Build history of the part. All positions in model axes, mm. A direction names the side the tool comes from. Coordinates: 2 decimals unless noted, no trailing zeros. Order: outer loops, then holes, each group sorted by start corner. A loop starts at its lowest first (then second) coordinate and runs counter-clockwise, first axis right, second up. Notation, with made-up numbers: M 40,-33 L 65,-33 A18 ccw 65,-28 Z; hole C -38,-22.5 d11. An arc over 180 degrees is marked long. Write item = value, one per line. Start each with the question number.
Q1. Band-saw the part on C-C on y = 1.25. Write the cut outline in (x, z), plus the area to 3 significant figures.
Q2. Drill centre lines: probe 1 along Y at (x, z) = (-3, 21); probe 2 along Z at (x, y) = (-7, -0.5); probe 3 along X at (y, z) = (18.5, 4). Where is each one in solid material? Low to high.
Q3. Pull direction X, two halves, no side cores. Call faces 5 (the face through (6.73, 18.1, 27.31)), 6 (the face through (12.626, 11, -5)), 7 (the face through (3, -4.786, 8)), 8 (the face through (-7.574, 8, 8)): released by +X, released by -X, zero draft, split by the parting line, or undercut.
Q4. Band-saw the part on B-B on z = 23. Write the cut outline in (x, y).
Q5. 3-axis set-ups, long thin cutter, end or side, ignore diameter. For faces 1 (the face through (3, -6.786, -1)), 2 (the face through (9, 6.958, 22)), 3 (the face through (13.626, 8, 8)), 4 (the face through (-0.95, 18.09, 27.31)): which of +Z, -Z, +X, -X, +Y, -Y reach the whole face in a straight line?
Q6. Pin check, flat tips, straight feed: P1, Ø5.5, axis at y = 6.5, z = -4.5, coming from the +X side; P2, Ø5, axis at x = 8, z = 10.5, coming from the +Y side; P3, Ø2, axis at y = -2.5, z = 14, coming from the +X side; P4, Ø1.1, axis at y = 18.5, z = 22, coming from the -X side. Stop position of each tip, or through.
Q7. Band-saw the part on D-D on x = 5.25. Write the cut outline in (y, z).
Q8. Band-saw the part on A-A on x = -3. Write the cut outline in (y, z), plus the area to 3 significant figures.
Autodesk Inventor part; units mm, degrees
ref_plane "Płaszczyzna konstrukcyjna1" through (12.6265, -6.7865, 0) normal (1, 0, 0) x (0, 0, -1)
ref_plane "YZ Plane" through (0, 0, 0) normal (1, 0, 0) x (0, 1, 0)
ref_plane "XZ Plane" through (0, 0, 0) normal (0, 1, 0) x (-1, 0, 0)
sketch "Szkic1" plane through (0, 0, 0) normal (0, 0, 1) x (1, 0, 0)
  line L0 (-7.5735, 20.8135) -> (13.6265, 20.8135)
  line L1 (13.6265, 20.8135) -> (13.6265, -4.7865)
  line L2 (13.6265, -4.7865) -> (-7.5735, -4.7865)
  line L3 (-7.5735, -4.7865) -> (-7.5735, 20.8135)
  line L4 (-9.5735, 22.8135) -> (15.6265, 22.8135)
  line L5 (15.6265, 22.8135) -> (15.6265, -6.7865)
  line L6 (15.6265, -6.7865) -> (-9.5735, -6.7865)
  line L7 (-9.5735, -6.7865) -> (-9.5735, 22.8135)
  point P0 (0, 0)
  dimension "d0" = 21.2
  dimension "d1" = 25.6
  dimension "d2" = 2
extrude "Wyciągnięcie proste1" add sketch "Szkic1" along normal blind 16.3 contours L0 L1 L2 L3
extrude "Wyciągnięcie proste2" add sketch "Szkic1" against normal blind 2 contours L0 L1 L2 L3 | L4 L5 L6 L7
ref_plane "Płaszczyzna konstrukcyjna1" through (12.6265, -6.7865, 0) normal (1, 0, 0) x (0, 0, -1)
sketch "Szkic2" plane through (12.6265, -6.7865, 0) normal (1, 0, 0) x (0, 0, -1)
  line L0 (2, 0) -> (2, 29.6)
  line L1 (0, 0) -> (2, 0)
  line L2 (0, 29.6) -> (2, 29.6)
  line L3 (0, 27.6) -> (-16.3, 27.6)
  line L4 (0, 2) -> (-16.3, 2)
  arc A0 (9, 19.6) -> (2, 26.6) centre (-7.5761, 10.0239) ccw
  line L5 (9, 19.6) -> (2, 3)
  point P0 (0, 6.7865)
  dimension "d8" = 7
  dimension "d9" = 29.6
  dimension "d10" = 2
  dimension "d11" = 10
  dimension "d12" = 1
  dimension "d13" = 1
extrude "Wyciągnięcie proste3" add sketch "Szkic2" against normal blind 18.7
sketch "Szkic3" plane through (0, 0, 16.3) normal (0, 0, 1) x (1, 0, 0)
  line L0 (13.6265, 20.8135) -> (-7.5735, 20.8135)
  line L1 (-7.5735, 20.8135) -> (-7.5735, -4.7865)
  line L2 (-7.5735, -4.7865) -> (13.6265, -4.7865)
  line L3 (13.6265, -4.7865) -> (13.6265, 20.8135)
  line L4 (-5.9377, 18.5947) -> (0.0623, 18.5947)
  line L5 (0.0623, 18.5947) -> (0.0623, 17.5947)
  line L6 (0.0623, 17.5947) -> (-5.9377, 17.5947)
  line L7 (-5.9377, 17.5947) -> (-5.9377, 18.5947)
  line L8 (5.7192, 18.5947) -> (11.7192, 18.5947)
  line L9 (11.7192, 18.5947) -> (11.7192, 17.5947)
  line L10 (11.7192, 17.5947) -> (5.7192, 17.5947)
  line L11 (5.7192, 17.5947) -> (5.7192, 18.5947)
  line L12 (-5.9377, 7.9577) -> (0.0623, 7.9577)
  line L13 (0.0623, 7.9577) -> (0.0623, 6.9577)
  line L14 (0.0623, 6.9577) -> (-5.9377, 6.9577)
  line L15 (-5.9377, 6.9577) -> (-5.9377, 7.9577)
  line L16 (5.7192, 7.9577) -> (11.7192, 7.9577)
  line L17 (11.7192, 7.9577) -> (11.7192, 6.9577)
  line L18 (11.7192, 6.9577) -> (5.7192, 6.9577)
  line L19 (5.7192, 6.9577) -> (5.7192, 7.9577)
  point P0 (0, 0)
  dimension "d16" = 6
  dimension "d17" = 1
  dimension "d18" = 6
  dimension "d19" = 1
  dimension "d20" = 6
  dimension "d21" = 1
  dimension "d22" = 6
  dimension "d23" = 1
extrude "Wyciągnięcie proste4" add sketch "Szkic3" along normal blind 12 contours L4 L5 L6 L7 | L8 L9 L10 L11 | L12 L13 L14 L15 | L16 L17 L18 L19
chamfer "Faza1" distance 2 angle 45 8 edges at (0.0623, 18.0947, 28.3) (-5.9377, 18.0947, 28.3) (11.7192, 18.0947, 28.3) (5.7192, 18.0947, 28.3) (11.7192, 7.4577, 28.3) (5.7192, 7.4577, 28.3) (0.0623, 7.4577, 28.3) (-5.9377, 7.4577, 28.3)
sketch "Szkic4" plane through (12.6265, -3.7865, -2) normal (0, -0.3886, -0.9214) x (-1, 0, 0)
  line L0 (6.8473, 17.5297) -> (14.0234, 17.5297) construction
  line L1 (14.0234, 17.5297) -> (14.0234, 9.4771) construction
  line L2 (14.0234, 9.4771) -> (6.8473, 9.4771) construction
  line L3 (6.8473, 9.4771) -> (6.8473, 17.5297) construction
  line L4 (8.3846, 8.6266) -> (9.6316, 8.6266) construction
  line L5 (9.6316, 8.6266) -> (9.6316, 4.3438) construction
  line L6 (9.6316, 4.3438) -> (8.3846, 4.3438) construction
  line L7 (8.3846, 4.3438) -> (8.3846, 8.6266) construction
properties part number "COTS_GENERIC_AC_Power_Switch_10A"
Recorded:
q1.outline = M -9.57,-2 L -6.07,-2 L -6.07,-4.12 L 12.63,-4.12 L 12.63,-2 L 15.63,-2 L 15.63,0 L 13.63,0 L 13.63,16.3 L -7.57,16.3 L -7.57,0 L -9.57,0 Z
q1.area = 436 mm2
q2.probe_1 = 6.96 to 7.96, 17.59 to 18.59
q2.probe_2 = -2 to 16.3
q2.probe_3 = -7.57 to 13.63
q3.face_5 = undercut
q3.face_6 = released by +X
q3.face_7 = zero draft
q3.face_8 = released by -X
q4.outline = M -5.94,6.96 L 0.06,6.96 L 0.06,7.96 L -5.94,7.96 Z; M -5.94,17.59 L 0.06,17.59 L 0.06,18.59 L -5.94,18.59 Z; M 5.72,6.96 L 11.72,6.96 L 11.72,7.96 L 5.72,7.96 Z; M 5.72,17.59 L 11.72,17.59 L 11.72,18.59 L 5.72,18.59 Z
q5.face_1 = +Z, -Z, +X, -X, -Y
q5.face_2 = +Z, +X, -X, -Y
q5.face_3 = +Z, +X, +Y, -Y
q5.face_4 = +Z, +Y, -Y
q6.P1 = 15.63
q6.P2 = 20.81
q6.P3 = 13.63
q6.P4 = -5.94
q7.outline = M -6.79,-2 L -3.79,-2 L 12.81,-9 A19.14 ccw 19.81,-2 L 22.81,-2 L 22.81,0 L 20.81,0 L 20.81,16.3 L -4.79,16.3 L -4.79,0 L -6.79,0 Z
q8.outline = M -6.79,-2 L -3.79,-2 L 12.81,-9 A19.14 ccw 19.81,-2 L 22.81,-2 L 22.81,0 L 20.81,0 L 20.81,16.3 L 18.59,16.3 L 18.59,28.3 L 17.59,28.3 L 17.59,16.3 L 7.96,16.3 L 7.96,28.3 L 6.96,28.3 L 6.96,16.3 L -4.79,16.3 L -4.79,0 L -6.79,0 Z
q8.area = 587 mm2
